Geometry: final body of the model. Coordinates: model frame, mm. Face numbers are marked on the shaded views. A direction names the side the tool comes from. Coordinates: 2 decimals unless noted, no trailing zeros. Loops run counter-clockwise (first coordinate to the right, second up) from the corner with the lowest first, then second, coordinate; pieces in that order, holes last. Notation, with made-up numbers: (-28, 27) - (6, 27) arc R9 ccw to (6, 43) - close; hole circle Ø9 at (65, 24). An arc over 180 degrees is marked (long way). Return JSON: item names as keys, results as strings.
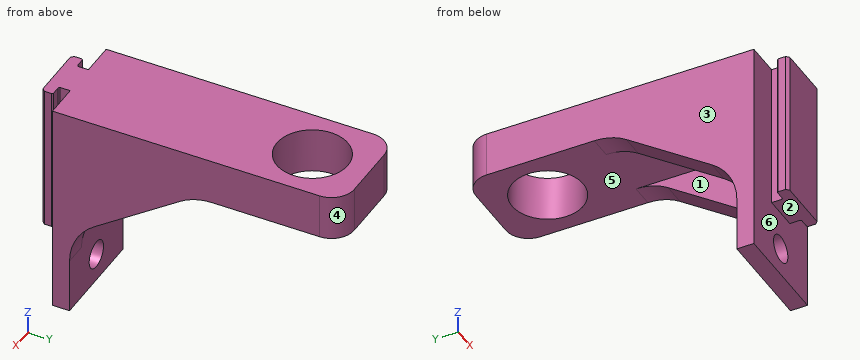
from build123d import *

# Parameters (mm, degrees)
EXTRUDE_1_DEPTH      = 4
EXTRUDE_1_DEPTH_BACK = 4
SKETCH_1_R           = 6.25
EXTRUDE_2_DEPTH      = 34
RIB_1_REACH          = 74.118
SKETCH_2_WALL_W      = 172.862971768
SKETCH_2_WALL_H      = 4
FILLET_1_R           = 10
EXTRUDE_3_DEPTH      = 22
CHAMFER_1_SIZE       = 0.2
SKETCH_4_R           = 2.4
CUT_EXTRUDE_1_DEPTH  = 60.506302187


with BuildPart() as part:
    # 草图1 → 凸台-拉伸1 (new, two sides: drawn at the far end of the back side and taken through both)
    # profile 1 of 3: a face of its own
    with BuildSketch(Plane.XY.offset(-EXTRUDE_1_DEPTH_BACK)):
        Polygon((-9, 10), (-3.05, 10), (3.05, 10), (9, 10), (9, 13), (-9, 13), align=None)
    # profile 2 of 3: a face of its own
    with BuildSketch(Plane.XY.offset(-EXTRUDE_1_DEPTH_BACK)):
        Polygon((3.05, 10), (-3.05, 10), (-3.05, 8), (-5.05, 8), (-5.05, 6.5), (-4.55, 6), (4.55, 6), (5.05, 6.5), (5.05, 8), (3.05, 8), align=None)
    # profile 3 of 3: a face of its own
    with BuildSketch(Plane.XY.offset(-EXTRUDE_1_DEPTH_BACK)):
        with BuildLine():
            Line((-9, 57), (-9, 13))
            Line((-9, 13), (9, 13))
            Line((9, 13), (9, 57))
            ThreePointArc((9, 57), (7.828427125, 59.828427125), (5, 61))
            Line((5, 61), (-5, 61))
            ThreePointArc((-5, 61), (-7.828427125, 59.828427125), (-9, 57))
        make_face()
        with Locations((0, 51)):
            Circle(SKETCH_1_R, mode=Mode.SUBTRACT)
    extrude(amount=EXTRUDE_1_DEPTH + EXTRUDE_1_DEPTH_BACK)

    # 草图1<6> → 凸台-拉伸2 (add)
    with BuildSketch(Plane.XY):
        Polygon((-9, 10), (-3.05, 10), (3.05, 10), (9, 10), (9, 13), (-9, 13), align=None)
    extrude(amount=-EXTRUDE_2_DEPTH)

    # 草图2 wall → 筋1 (add, up to next)
    with BuildSketch(Plane(origin=(9, 24, -11.5), x_dir=(0, -0.826227342808, -0.563336824642), z_dir=(0, 0.563336824642, -0.826227342808)), mode=Mode.PRIVATE) as rib_1_sk1:
        with Locations((0, 2)):
            Rectangle(SKETCH_2_WALL_W, SKETCH_2_WALL_H)
    rib_1_tool1 = extrude(rib_1_sk1.sketch, amount=-RIB_1_REACH, mode=Mode.PRIVATE) - part.part
    rib_1 = rib_1_tool1.solids().sort_by_distance((9, 24, -11.5))[0]
    add(rib_1)

    # 镜向1: 筋1 across plane
    add(rib_1.mirror(Plane(origin=(0, 0, 0), x_dir=(0, 0, 1), z_dir=(1, 0, 0))))

    # 圆角1
    fillet_1_edges = [part.edges().sort_by_distance(p)[0] for p in [
        (7, 13, -19),
        (7, 35, -4),
        (-7, 13, -19),
        (-7, 35, -4),
    ]]
    fillet(fillet_1_edges, radius=FILLET_1_R)

    # 草图1<7> → 凸台-拉伸3 (add)
    with BuildSketch(Plane.XY):
        Polygon((3.05, 8), (5.05, 8), (5.05, 6.5), (4.55, 6), (-4.55, 6), (-5.05, 6.5), (-5.05, 8), (-3.05, 8), (-3.05, 10), (3.05, 10), align=None)
    extrude(amount=-EXTRUDE_3_DEPTH)

    # 倒角1
    chamfer_1_edges = [part.edges().sort_by_distance(p)[0] for p in [
        (5.05, 8, -9),
        (-5.05, 8, -9),
        (-3.05, 8, -9),
        (3.05, 8, -9),
    ]]
    chamfer(chamfer_1_edges, length=CHAMFER_1_SIZE)

    # 草图4 → 切除-拉伸1 (cut, through all)
    with BuildSketch(Plane(origin=(0, 13, 0), x_dir=(1, 0, 0), z_dir=(0, 1, 0))):
        with Locations(Location((0, 29, 0), (0, 0, 270))):
            Circle(SKETCH_4_R)
    extrude(amount=-CUT_EXTRUDE_1_DEPTH, mode=Mode.SUBTRACT)


solid = part.part
Item 1: Section query A-A, the plane z = -29. Return loops of the section in (x, y), and give its area (3 significant figures).
Worked out:
{"outline": "(-9, 10) - (-2.4, 10) - (-2.4, 13) - (-9, 13) - close; (2.4, 10) - (9, 10) - (9, 13) - (2.4, 13) - close", "area": "39.6 mm^2"}
Item 2: First-contact query: pin 1 Ø0.8 at (x, z) = (4, -9.5) entering from +Y; pin 2 Ø6 at (y, z) = (28.5, -15) entering from +X; pin 3 Ø1 at (x, y) = (6.5, 21) entering from -Z; pin 4 Ø1.4 at (y, z) = (7, -10.5) entering from -X. Flat tips, straight axial feed; report the tip coordinate or a pass-through.
Worked out:
{"pin 1": "y = 13", "pin 2": "through", "pin 3": "z = -13.89", "pin 4": "x = -5.05"}
Item 3: Section query C-C, the plane x = 0. Return loops of the section in (y, z), and give its area (3 significant figures).
Worked out:
{"outline": "(6, -22) - (10, -22) - (10, -26.6) - (13, -26.6) - (13, -4) - (44.75, -4) - (44.75, 4) - (6, 4) - close; (10, -34) - (13, -34) - (13, -31.4) - (10, -31.4) - close; (57.25, -4) - (61, -4) - (61, 4) - (57.25, 4) - close", "area": "488 mm^2"}
Item 4: Ray query, probe 1 along Y at (x, z) = (0, 2); probe 2 along Y at (x, z) = (-3.25, -21); probe 3 along Y at (x, z) = (1.5, -24). Return the intervals inside material, ascending. Write a range as from..to.
Worked out:
{"probe 1": "6..44.75, 57.25..61", "probe 2": "6..8, 10..13", "probe 3": "10..13"}
Item 5: Section query D-D, the plane y = 18. Return loops of the section in (x, z), and give its area (3 significant figures).
Worked out:
{"outline": "(-9, -15.59) - (-5, -15.59) - (-5, -4) - (5, -4) - (5, -15.59) - (9, -15.59) - (9, 4) - (-9, 4) - close", "area": "237 mm^2"}
Item 6: Section query B-B, the plane y = 51. Return loops of the section in (x, z), and give its area (3 significant figures).
Worked out:
{"outline": "(-9, -4) - (-6.25, -4) - (-6.25, 4) - (-9, 4) - close; (6.25, -4) - (9, -4) - (9, 4) - (6.25, 4) - close", "area": "44.0 mm^2"}
Item 7: Reachability of the marked faces 1, 2 and 3 from +Z, -Z, +X, -X, +Y, -Y: full face, straight path, thin tool, end or side. Return the list, or none.
Worked out:
{"face 1": "-Z, +Y", "face 2": "-Z, +X, -X, -Y", "face 3": "+Z, -Z, -X, +Y, -Y"}
Item 8: Mould query, pull axis X, two halves, no side actions, for the marked faces 4, 5 and 6. Classes: +X half, -X half, draft (parallel to the pull), parting line (faces both ways), or undercut.
Worked out:
{"face 4": "+X half", "face 5": "undercut", "face 6": "draft"}
